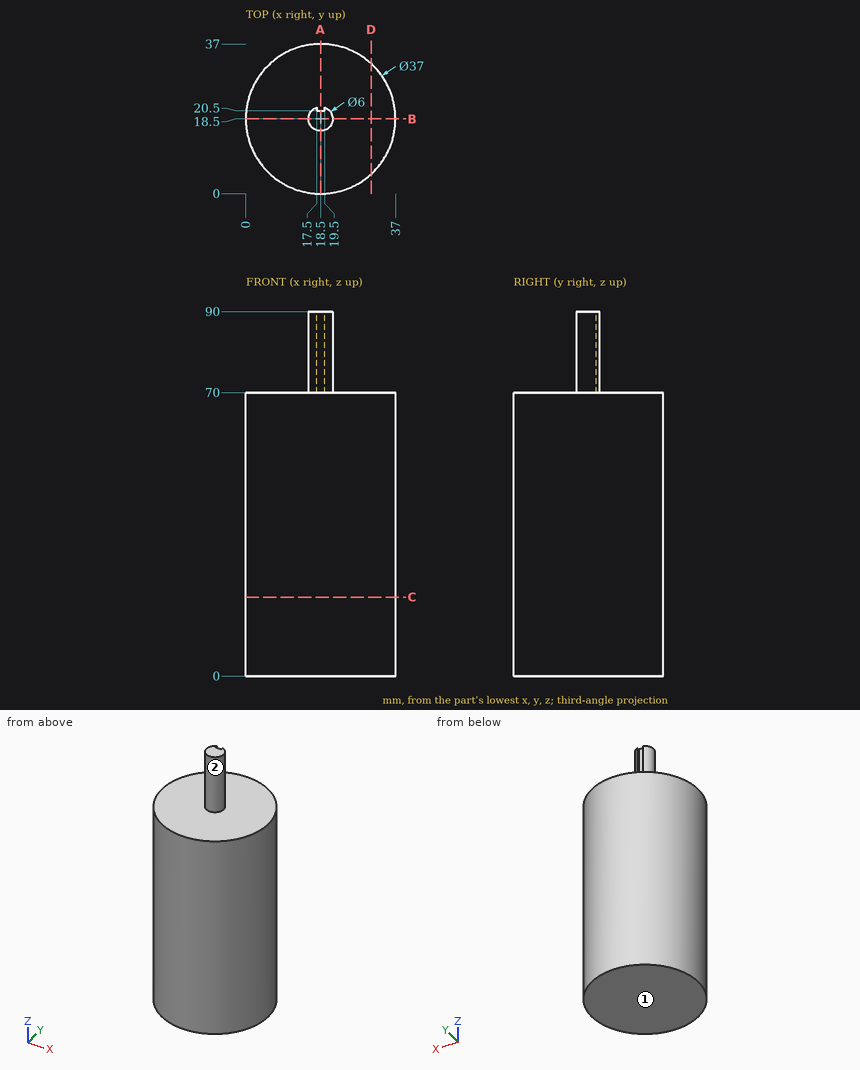
Source: three-view drawing plus pictorial views. Frame: mm from the lowest corner of the part. A direction names the side the tool comes from. Coordinates: 2 decimals unless noted, no trailing zeros. Loops run counter-clockwise (first coordinate to the right, second up) from the corner with the lowest first, then second, coordinate; pieces in that order, holes last. Notation, with made-up numbers: (59.25, 54) -> (64.25, 54) arc R17 cw to (64.25, 67) -> close; hole circle Ø2 at (16.25, 76.25). An arc over 180 degrees is marked (long way). Answer in a Markdown table with one row per item. Add a question column.
Q1. Ray query, line 1 along Z through (x, y) = (10, 2.5); line 2 along X through (y, z) = (18, 10.5). Return the intervals inside material, ascending.
Q2. Reachability of the marked faces 1 and 2 from +Z, -Z, +X, -X, +Y, -Y: full face, straight path, thin tool, end or side. Return the list, or none.
Q3. Section C-C on z = 19.5. Return the cut outline in (x, y).
Q4. Section A-A on x = 18.5. Return the cut outline in (y, z), and give its area (3 significant figures).
Q5. Section B-B on y = 18.5. Return the cut outline in (x, z), and give its area (3 significant figures).
Q6. Section D-D on x = 31. Return the cut outline in (y, z), and give its area (3 significant figures).
Q7. Contact query for flat-ended pins moving along their axis: pin 1 Ø8 at (y, z) = (23, 68) entering from +X; pin 2 Ø6 at (x, y) = (19.5, 18) entering from -Z; pin 3 Ø8 at (y, z) = (5.5, 46) entering from -X; pin 4 Ø10 at (x, z) = (18, 17.5) entering from +Y. Output: stop coordinate, or through.
Computed values:
| question | item | result |
|---|---|---|
| 1 | line 1 | z = 0 to 70 |
| 1 | line 2 | x = 0.01 to 36.99 |
| 2 | face 1 | -Z, +X, -X, +Y, -Y |
| 2 | face 2 | +Z |
| 3 | outline | circle Ø37 at (18.5, 18.5) |
| 4 | outline | (0, 0) -> (37, 0) -> (37, 70) -> (20.5, 70) -> (20.5, 90) -> (15.5, 90) -> (15.5, 70) -> (0, 70) -> close |
| 4 | area | 2,690 mm^2 |
| 5 | outline | (0, 0) -> (37, 0) -> (37, 70) -> (21.5, 70) -> (21.5, 90) -> (15.5, 90) -> (15.5, 70) -> (0, 70) -> close |
| 5 | area | 2,710 mm^2 |
| 6 | outline | (4.86, 0) -> (32.14, 0) -> (32.14, 70) -> (4.86, 70) -> close |
| 6 | area | 1,910 mm^2 |
| 7 | pin 1 | stops at x = 36.99 |
| 7 | pin 2 | stops at z = 0 |
| 7 | pin 3 | stops at x = 2.34 |
| 7 | pin 4 | stops at y = 37 |
